Check sheet for the modelled part. Datum: model origin and axes. Units: mm. A direction names the side the tool comes from. Give positions to 0.01 mm unless a question says otherwise; leave off trailing zeros. Loops run counter-clockwise (first coordinate to the right, second up) from the corner with the lowest first, then second, coordinate; pieces in that order, holes last. Notation, with made-up numbers: (-13.5, 74) -> (3.5, 74) arc R21 ccw to (3.5, 85) -> close; hole circle Ø10 at (-26, 27). An arc over 180 degrees is marked (long way). Write each question's results on one line, items separated by ' | '. Start each with the question number.
1. Gauge pin test, flat ends, axial feed: pin 1 Ø6 at (x, y) = (-8, -6.5) entering from +Z; pin 2 Ø3.5 at (y, z) = (-7.77, 19.25) entering from -X; pin 3 Ø2.5 at (y, z) = (-7.77, -40.75) entering from +X; pin 4 Ø2.5 at (y, z) = (-7.77, -120.75) entering from -X. Record the tip position at first contact, or that the pin passes through.
2. Material ranges on L1, parallel to X at y = -10.5, z = -124; L2, parallel to X at y = -2.5, z = -129.5; L3, parallel to Z at x = -8, y = -1.25, recorded low to high. Write a range as from..to.
3. Cross-section at A-A on z = -112.5. Record the boundary of the cut face in (x, y).
4. Cross-section at B-B on y = -3. Record the boundary of the cut face in (x, z).
5. Tool access check on faces 1 (the face through (15.831, -7, -49)), 2 (the face through (17.31, -7.078, -99.415)), 3 (the face through (-19, -15, -60)). Record the directions out of +Z, -Z, +X, -X, +Y, -Y that give a thin tool (end or side, any length) a straight path to the whole face; none if there is none.
6. Mould release check, pull along X, two halves, no side actions. Record for faces 4 (the face through (-0.8, -7.4, -145.41)), 5 (the face through (-21.169, -7, -49)), 6 (the face through (17, -7, 28.586)), 7 (the face through (-18.169, -7, -51)): +X half, -X half, draft (parallel to the pull), parting line (faces both ways), or undercut.
7. Cross-section at D-D on x = 10. Record the boundary of the cut face in (y, z), and give its area (3 significant figures).
8. Cross-section at C-C on x = -8.5. Record the boundary of the cut face in (y, z).
from build123d import *

# Parameters (mm, degrees)
F1_DEPTH = 15
F3_D     = 3
F3_DEPTH = 18.8319625536
F4_D     = 3


# Not quite as in the source:
# - a feature names something its author has since deleted; it is built from what else it names


with BuildPart() as f1:
    # F0 (on Front) → F1 (new body)
    with BuildSketch(Plane.XZ):
        with BuildLine():
            Line((-18.1690374464, 28.586239934), (-21.1690374464, 28.586239934))
            Line((-21.1690374464, 28.586239934), (-21.1690374464, -128.413760066))
            ThreePointArc((-21.1690374464, -128.413760066), (-1.1690374464, -148.413760066), (18.8309625536, -128.413760066))
            Line((18.8309625536, -128.413760066), (18.8309625536, 28.586239934))
            Line((18.8309625536, 28.586239934), (15.8309625536, 28.586239934))
            Line((15.8309625536, 28.586239934), (15.8309625536, -128.413760066))
            ThreePointArc((15.8309625536, -128.413760066), (-1.1690374464, -145.413760066), (-18.1690374464, -128.413760066))
            Line((-18.1690374464, -128.413760066), (-18.1690374464, 28.586239934))
        make_face()
    extrude(amount=F1_DEPTH)

    # F3 (through all, one way)
    with BuildSketch(Plane(origin=(0, 0, 0), x_dir=(0, 1, 0), z_dir=(-1, 0, 0))):
        with Locations((-7.7703874558, 0.7461506128), (-7.7703874558, 20.7461506128), (-7.7703874558, 40.7461506128), (-7.7703874558, 60.7461506128), (-7.7703874558, 80.7461506128), (-7.7703874558, 100.7461506128), (-7.7703874558, 120.7461506128), (-7.7703874558, -19.2538493872)):
            Circle(F3_D / 2)
    extrude(amount=-F3_DEPTH, mode=Mode.SUBTRACT)

    # F4 (through all)
    with Locations(Plane.YZ):
        with Locations((-7.7703874558, 19.2538493872), (-7.7703874558, -120.7461506128)):
            Hole(F4_D / 2)


solid = f1.part
Geometry says:
1) pin 1: z = -142.28 | pin 2: x = -21.17 | pin 3: x = -18.17 | pin 4: through
2) L1: -21.17..-18.17, 15.83..18.83 | L2: -21.14..-18.13, 15.8..18.8 | L3: -147.21..-143.98
3) outline: (-21.17, -15) -> (-18.17, -15) -> (-18.17, 0) -> (-21.17, 0) -> close; (15.83, -15) -> (18.83, -15) -> (18.83, 0) -> (15.83, 0) -> close
4) outline: (-21.17, -128.41) arc R20 ccw to (18.83, -128.41) -> (18.83, 28.59) -> (15.83, 28.59) -> (15.83, -128.41) arc R17 cw to (-18.17, -128.41) -> (-18.17, 28.59) -> (-21.17, 28.59) -> close
5) face 1: +Z, +Y, -Y | face 2: +X | face 3: +Z, -Z, +X, -X, -Y
6) face 4: undercut | face 5: -X half | face 6: draft | face 7: undercut
7) outline: (-15, -145) -> (0, -145) -> (0, -141.23) -> (-15, -141.23) -> close | area: 56.6 mm^2
8) outline: (-15, -147.02) -> (0, -147.02) -> (0, -143.75) -> (-15, -143.75) -> close
